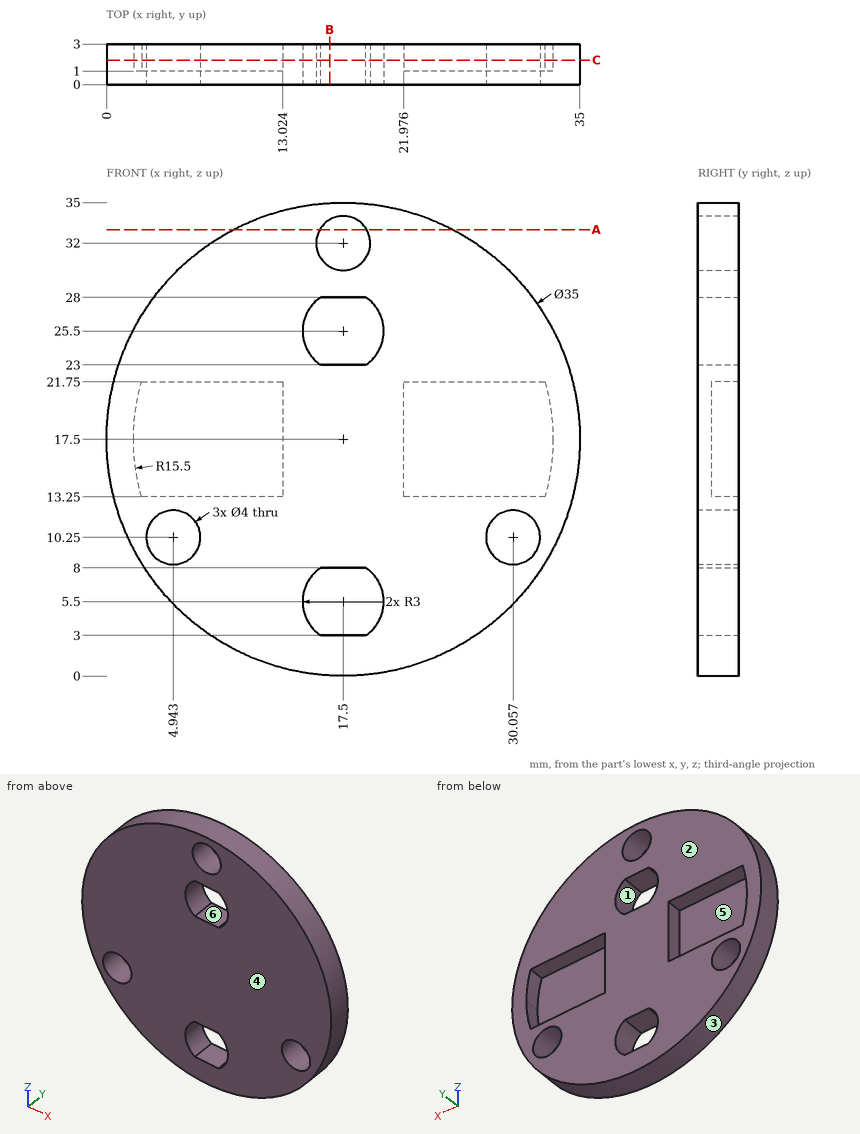
Geometry check sheet. Reference: drawing and pictorial views, mm from the part's lowest x, y, z. A direction names the side the tool comes from. Coordinates: 2 decimals unless noted, no trailing zeros. Order: outer loops, then holes, each group sorted by start corner. A loop starts at its lowest first (then second) coordinate and runs counter-clockwise, first axis right, second up. Notation, with made-up numbers: (-30.75, -37.5) -> (-7.75, -37.5) arc R32 ccw to (-7.75, 1.5) -> close; hole circle Ø6 at (59, 17). An arc over 180 degrees is marked (long way). Write item = value, one per line. Start each with the question number.
1) Go/stop test with flat-tipped pins: P1, Ø7, axis at x = 28.5, z = 18, coming from the +Y side; P2, Ø0.6, axis at x = 25.5, y = 2.5, coming from the +Z side (1 decimal); P3, Ø1.5, axis at x = 31.5, y = 2.5, coming from the -Z side; P4, Ø2.5, axis at x = 17.5, z = 32, coming from the +Y side. Record where each tip stops, or that it passes through.
2) Access from +Z, -Z, +X, -X, +Y, -Y to the whole of each face (thin tool, end or side, straight path). Record for the marked faces 4, 5 and 6.
3) Cross-section at A-A (z = 33). Enter the section's corners in (x, y).
4) Mould release check, pull along Z, two halves, no side actions. Record for the marked faces 1, 2 and 3: +Z half, -Z half, draft (parallel to the pull), parting line (faces both ways), or undercut.
5) Material ranges on L1, parallel to X at y = 2.5, z = 18; L2, parallel to X at y = 1.65, z = 10.25; L3, parallel to Z at x = 16, y = 2.45 (1 decimal), recorded low to high.
6) Cross-section at C-C (y = 1.8). Enter the section's corners in (x, z).
7) Cross-section at B-B (x = 16.5). Enter the section's corners in (y, z).
Ans:
q1.P1 = 1
q1.P2 = 33.2
q1.P3 = 6.07
q1.P4 = through
q2.face_4 = +Z, -Z, +X, -X, -Y
q2.face_5 = +Y
q2.face_6 = +Y, -Y
q3.outline = (9.38, 0) -> (15.77, 0) -> (15.77, 3) -> (9.38, 3) -> close; (19.23, 0) -> (25.62, 0) -> (25.62, 3) -> (19.23, 3) -> close
q4.face_1 = undercut
q4.face_2 = draft
q4.face_3 = parting line
q5.L1 = 0.01 to 2.01, 13.02 to 21.98, 32.99 to 34.99
q5.L2 = 1.57 to 2.94, 6.94 to 28.06, 32.06 to 33.43
q5.L3 = 0.1 to 3, 8 to 23, 28 to 30.7, 33.3 to 34.9
q6.outline = circle Ø35 at (17.5, 17.5); hole (2.59, 13.25) -> (13.02, 13.25) -> (13.02, 21.75) -> (2.59, 21.75) arc R15.5 ccw to start; hole circle Ø4 at (4.94, 10.25); hole circle Ø4 at (17.5, 32); hole (15.84, 3) -> (19.16, 3) arc R3 ccw to (19.16, 8) -> (15.84, 8) arc R3 ccw to start; hole (15.84, 23) -> (19.16, 23) arc R3 ccw to (19.16, 28) -> (15.84, 28) arc R3 ccw to start; hole (21.98, 13.25) -> (32.41, 13.25) arc R15.5 ccw to (32.41, 21.75) -> (21.98, 21.75) -> close; hole circle Ø4 at (30.06, 10.25)
q7.outline = (0, 0.03) -> (3, 0.03) -> (3, 3) -> (0, 3) -> close; (0, 8) -> (3, 8) -> (3, 23) -> (0, 23) -> close; (0, 28) -> (3, 28) -> (3, 30.27) -> (0, 30.27) -> close; (0, 33.73) -> (3, 33.73) -> (3, 34.97) -> (0, 34.97) -> close
